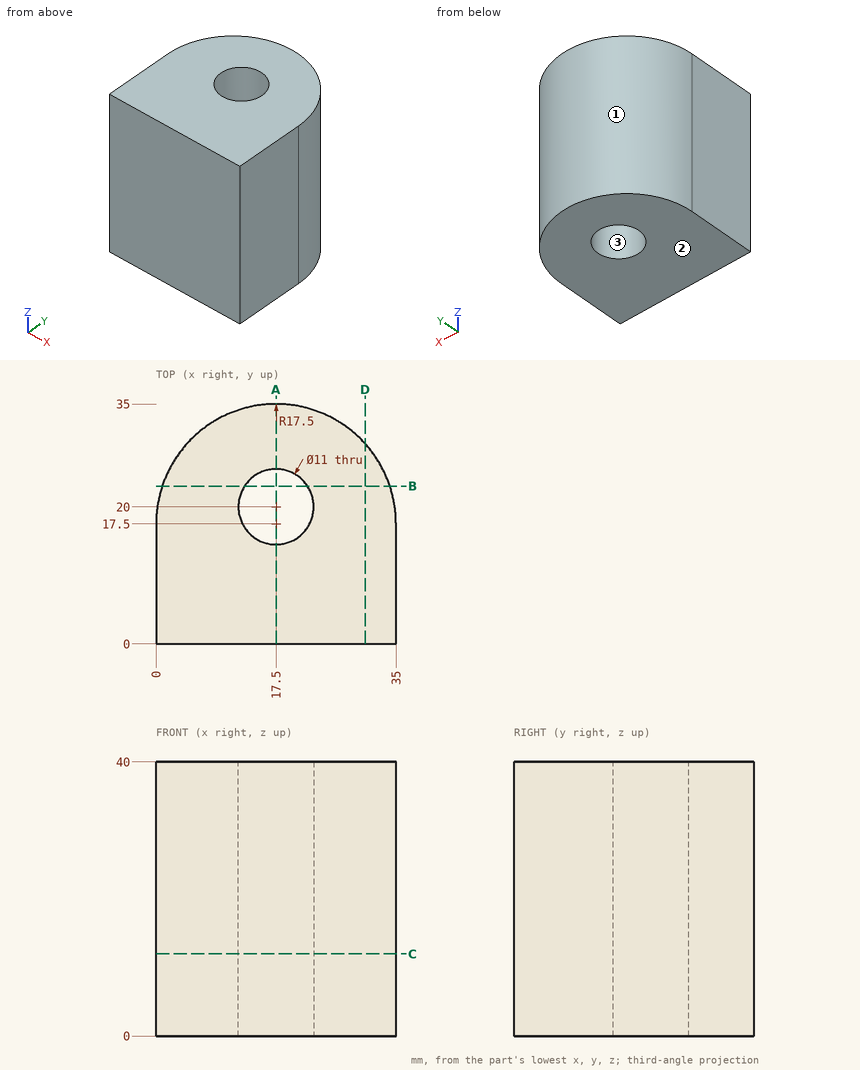
Geometry: see drawing. Coordinates: mm, zero at the bounding-box minimum. Give positions to 0.01 mm unless a question says otherwise; leave off trailing zeros. Order: outer loops, then holes, each group sorted by start corner. A loop starts at its lowest first (then second) coordinate and runs counter-clockwise, first axis right, second up.
Q1. Draft query along Y for the marked faces 1, 2 and 3. Return one class per face: +Y half, -Y half, draft (parallel to the pull), parting line (faces both ways), or undercut.
Checked values:
face 1: +Y half
face 2: draft
face 3: undercut
Q2. Section B-B on y = 23. Output: boundary loops of the cut face in (x, z), and give its area (3 significant figures).
Checked values:
outline: (0.89, 0) - (12.89, 0) - (12.89, 40) - (0.89, 40) - close; (22.11, 0) - (34.11, 0) - (34.11, 40) - (22.11, 40) - close
area: 960 mm2
Q3. Section D-D on x = 30.5. Output: boundary loops of the cut face in (y, z).
Checked values:
outline: (0, 0) - (29.22, 0) - (29.22, 40) - (0, 40) - close
Q4. Contact query for flat-ended pins moving along their axis: pin 1 Ø3 at (y, z) = (31, 29.5) entering from +X; pin 2 Ø6 at (x, z) = (4, 5.5) entering from +Y. Output: stop coordinate, or through.
Checked values:
pin 1: stops at x = 30.24
pin 2: stops at y = 31.5
Q5. Section A-A on x = 17.5. Output: boundary loops of the cut face in (y, z), and give its area (3 significant figures).
Checked values:
outline: (0, 0) - (14.5, 0) - (14.5, 40) - (0, 40) - close; (25.5, 0) - (35, 0) - (35, 40) - (25.5, 40) - close
area: 960 mm2
Q6. Section C-C on z = 12. Output: boundary loops of the cut face in (x, y).
Checked values:
outline: (0, 0) - (35, 0) - (35, 17.5) arc R17.5 ccw to (0, 17.5) - close; hole circle Ø11 at (17.5, 20)
Q7. Ray query, probe 1 along Y at (x, z) = (17.5, 23); probe 2 along Y at (x, z) = (22, 15.5); probe 3 along X at (y, z) = (23.5, 36.5). Return the intervals inside material, ascending.
Checked values:
probe 1: y = 0 to 14.5, 25.5 to 35
probe 2: y = 0 to 16.84, 23.16 to 34.41
probe 3: x = 1.06 to 13.26, 21.74 to 33.94
